Check sheet for the modelled part. Datum: model origin and axes. Units: mm. Coordinates: 2 decimals unless noted, no trailing zeros. Order: outer loops, then holes, each group sorted by start corner. A loop starts at its lowest first (then second) coordinate and runs counter-clockwise, first axis right, second up.
1. Cross-section at A-A (x = 181.5). Enter the section's corners in (y, z) (3 decimals).
2. Cross-section at D-D (x = 33). Enter the section's corners in (y, z) (3 decimals), then the cut area to 3 significant figures.
3. Cross-section at C-C (y = 333.5). Enter the section's corners in (x, z) (3 decimals).
4. Gauge pin test, flat ends, axial feed: pin 1 Ø12 at (x, y) = (108.5, 159) entering from -Z; pin 2 Ø1 at (y, z) = (308, 2) entering from +X; pin 3 Ø1 at (y, z) = (343.5, 2) entering from +X. Record the tip position at first contact, or that the pin passes through.
5. Cross-section at B-B (z = 0.55). Enter the section's corners in (x, y) (3 decimals).
6. Thickness scan on line 1 (Y direction, x = 149.5, z = 2.3); line 2 (Y direction, x = 15, z = 2.3) (3 decimals); line 3 (X direction, y = 331.5, z = 1.95). Record the ranges inside material, lowest first.
Autodesk Inventor part; units mm, degrees
ref_plane "YZ Plane" through (0, 0, 0) normal (1, 0, 0) x (0, 1, 0)
ref_plane "XZ Plane" through (0, 0, 0) normal (0, 1, 0) x (-1, 0, 0)
ref_plane "XY Plane" through (0, 0, 0) normal (0, 0, 1) x (1, 0, 0)
sketch "Sketch1" plane through (0, 0, 0) normal (0, 0, 1) x (1, 0, 0)
  line L0 (0, 0) -> (203.2, 0)
  line L1 (203.2, 381) -> (0, 381)
  line L2 (203.2, 352.425) -> (177.8, 352.425)
  line L3 (177.8, 352.425) -> (177.8, 323.85)
  line L4 (177.8, 323.85) -> (146.05, 323.85)
  line L5 (146.05, 323.85) -> (146.05, 285.75)
  line L6 (146.05, 285.75) -> (177.8, 285.75)
  line L7 (177.8, 285.75) -> (177.8, 206.375)
  line L8 (177.8, 206.375) -> (203.2, 206.375)
  line L9 (0, 352.425) -> (25.4, 352.425)
  line L10 (25.4, 352.425) -> (25.4, 323.85)
  line L11 (25.4, 323.85) -> (57.15, 323.85)
  line L12 (57.15, 323.85) -> (57.15, 285.75)
  line L13 (57.15, 285.75) -> (25.4, 285.75)
  line L14 (25.4, 285.75) -> (25.4, 257.175)
  line L15 (25.4, 257.175) -> (0, 257.175)
  line L16 (203.2, 0) -> (203.2, 206.375)
  line L17 (203.2, 352.425) -> (203.2, 381)
  line L18 (0, 381) -> (0, 352.425)
  line L19 (0, 257.175) -> (0, 0)
  dimension "d0" = 203.2
  dimension "d1" = 381
  dimension "d4" = 25.4
  dimension "d5" = 28.575
  dimension "d6" = 31.75
  dimension "d7" = 38.1
  dimension "d8" = 79.375
  dimension "d9" = 28.575
  dimension "d10" = 25.4
  dimension "d11" = 28.575
  dimension "d12" = 31.75
  dimension "d13" = 38.1
  dimension "d14" = 31.75
  dimension "d15" = 28.575
  dimension "d16" = 28.575
extrude "Extrusion1" add sketch "Sketch1" along normal blind 3.175
properties part number "Collector Side" material "Polycarbonate, Clear"
Data:
1. outline: (0, 0) - (206.375, 0) - (206.375, 3.175) - (0, 3.175) - close; (352.425, 0) - (381, 0) - (381, 3.175) - (352.425, 3.175) - close
2. outline: (0, 0) - (285.75, 0) - (285.75, 3.175) - (0, 3.175) - close; (323.85, 0) - (381, 0) - (381, 3.175) - (323.85, 3.175) - close
2. area: 1,090 mm2
3. outline: (25.4, 0) - (177.8, 0) - (177.8, 3.175) - (25.4, 3.175) - close
4. pin 1: stops at z = 0
4. pin 2: stops at x = 146.05
4. pin 3: stops at x = 177.8
5. outline: (0, 0) - (203.2, 0) - (203.2, 206.375) - (177.8, 206.375) - (177.8, 285.75) - (146.05, 285.75) - (146.05, 323.85) - (177.8, 323.85) - (177.8, 352.425) - (203.2, 352.425) - (203.2, 381) - (0, 381) - (0, 352.425) - (25.4, 352.425) - (25.4, 323.85) - (57.15, 323.85) - (57.15, 285.75) - (25.4, 285.75) - (25.4, 257.175) - (0, 257.175) - close
6. line 1: y = 0 to 285.75, 323.85 to 381
6. line 2: y = 0 to 257.175, 352.425 to 381
6. line 3: x = 25.4 to 177.8
